Read the model definition and answer for the solid it produces. Units are mm, in the model's axes. Face numbers are marked on the shaded views. A direction names the side the tool comes from. Coordinates: 2 decimals unless noted, no trailing zeros. Loops run counter-clockwise (first coordinate to the right, second up) from the corner with the lowest first, then second, coordinate; pieces in that order, holes last. Notation, with made-up numbers: (22, 15.5) -> (59, 15.5) arc R17 cw to (59, 21.5) -> close; hole circle Ø6 at (0, 86.25). An arc over 180 degrees is marked (long way). Answer in a Markdown table with one row per item.
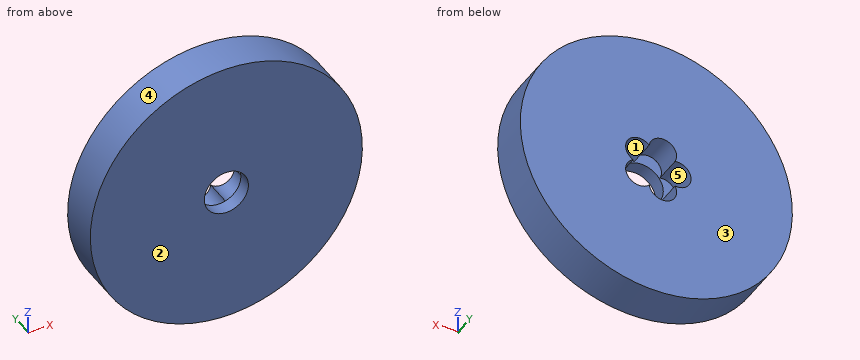
```python
from build123d import *

# Parameters (mm, degrees)
SKETCH1_R           = 92.5
BOSS_EXTRUDE1_DEPTH = 28
SKETCH2_R           = 15
CUT_EXTRUDE1_DEPTH  = 134.777800849
SKETCH3_R           = 9.366362932
CUT_EXTRUDE2_DEPTH  = 18.658456
CIRPATTERN1_START   = 9.341543819
CIRPATTERN1_DEPTH   = 18.658456181


# Read off the part's stored shape, not the designer's step: CirPattern1
with BuildPart() as part:
    # Sketch1 → Boss-Extrude1 (new body)
    with BuildSketch(Plane(origin=(0, 0, 0), x_dir=(1, 0, 0), z_dir=(0, 1, 0))):
        with Locations(Location((0, 0, 0), (0, 0, 270))):
            Circle(SKETCH1_R)
    extrude(amount=BOSS_EXTRUDE1_DEPTH)

    # Sketch2 → Cut-Extrude1 (cut, through all)
    with BuildSketch(Plane(origin=(0, 0, 0), x_dir=(1, 0, 0), z_dir=(0, 1, 0))):
        with Locations(Location((0, 0, 0), (0, 0, 270))):
            Circle(SKETCH2_R)
    extrude(amount=CUT_EXTRUDE1_DEPTH, mode=Mode.SUBTRACT)

    # Sketch3 → Cut-Extrude2 (cut)
    with BuildSketch(Plane(origin=(0, 28, 0), x_dir=(1, 0, 0), z_dir=(0, 1, 0))):
        with Locations((-14.249853525, 0)):
            Circle(SKETCH3_R)
    extrude(amount=-CUT_EXTRUDE2_DEPTH, mode=Mode.SUBTRACT)

    # CirPattern1 outline → CirPattern1 (cut)
    with BuildSketch(Plane(origin=(0, 0, 0), x_dir=(1, 0, 0), z_dir=(0, 1, 0)).offset(CIRPATTERN1_START)):
        with BuildLine():
            ThreePointArc((-11.941511199, -9.077461665), (-12.328101946, -9.167094711), (-12.718142529, -9.240271425))
            ThreePointArc((-12.718142529, -9.240271425), (-7.297812228, -22.460356552), (4.857898172, -14.951073231))
            ThreePointArc((4.857898172, -14.951073231), (19.105920457, -13.881263749), (15.720488714, 0))
            ThreePointArc((15.720488714, 0), (19.105920457, 13.881263749), (4.857898172, 14.951073231))
            ThreePointArc((4.857898172, 14.951073231), (-7.297812228, 22.460356552), (-12.718142529, 9.240271425))
            ThreePointArc((-12.718142529, 9.240271425), (-12.328101946, 9.167094711), (-11.941511199, 9.077461665))
            ThreePointArc((-11.941511199, 9.077461665), (15, 0), (-11.941511199, -9.077461665))
        make_face()
    extrude(amount=CIRPATTERN1_DEPTH, mode=Mode.SUBTRACT)


solid = part.part
```
1. A cutting plane is placed at A-A on x = 0. Give the vertices of the cut face in (y, z).
A:
| item | result |
|---|---|
| outline | (0, -92.5) -> (28, -92.5) -> (28, -21.82) -> (9.34, -21.82) -> (9.34, -15) -> (0, -15) -> close; (0, 15) -> (9.34, 15) -> (9.34, 21.82) -> (28, 21.82) -> (28, 92.5) -> (0, 92.5) -> close |
2. Find the intervals of material crossed by probe 1 along X at (y, z) = (4.25, 0); probe 2 along X at (y, z) = (13.5, 11); probe 3 along Z at (x, y) = (13, 9), in increasing order.
A:
| item | result |
|---|---|
| probe 1 | x = -92.5 to -15, 15 to 92.5 |
| probe 2 | x = -91.84 to -13.42, 20.52 to 91.84 |
| probe 3 | z = -91.58 to -7.48, 7.48 to 91.58 |
3. A tool of negligible diameter and unlimited length cuts with its end or side. For the marked faces 1 and 2, from which of +Z, -Z, +X, -X, +Y, -Y can it reach the whole face along a straight path? Write none if from no direction.
A:
| item | result |
|---|---|
| face 1 | +Y |
| face 2 | +Z, -Z, +X, -X, -Y |
4. A cutting plane is placed at B-B on z = -3. Give the vertices of the cut face in (x, y), and give its area (3 significant figures).
A:
| item | result |
|---|---|
| outline | (-92.45, 0) -> (-14.7, 0) -> (-14.7, 9.34) -> (-23.12, 9.34) -> (-23.12, 28) -> (-92.45, 28) -> close; (14.7, 0) -> (92.45, 0) -> (92.45, 28) -> (19.2, 28) -> (19.2, 9.34) -> (14.7, 9.34) -> close |
| area | 4,110 mm2 |
5. A cutting plane is placed at D-D on x = 57. Give the vertices of the cut face in (y, z), and give its area (3 significant figures).
A:
| item | result |
|---|---|
| outline | (0, -72.85) -> (28, -72.85) -> (28, 72.85) -> (0, 72.85) -> close |
| area | 4,080 mm2 |
6. The mould has two halves that part along X. Classify the marked faces 3, 4 and 5: pulls with the +X half, pulls with the -X half, needs draft (parallel to the pull), parting line crosses it, or undercut.
A:
| item | result |
|---|---|
| face 3 | needs draft |
| face 4 | parting line crosses it |
| face 5 | undercut |
7. Given pin 1 Ø5 at (x, y) = (-64.5, 12.5) entering from -Z; pin 2 Ø2 at (x, y) = (17.5, 13.5) entering from +Z; pin 3 Ø1 at (x, y) = (6, 11) entering from -Z, each flat-ended and moving along its own axis, determine where each tip first touches the part or whether it passes through.
A:
| item | result |
|---|---|
| pin 1 | stops at z = -68.65 |
| pin 2 | stops at z = 91.02 |
| pin 3 | stops at z = -92.34 |
8. A cutting plane is placed at C-C on y = 11.75. Give the vertices of the cut face in (x, z), and give its area (3 significant figures).
A:
| item | result |
|---|---|
| outline | circle Ø185 at (0, 0); hole (-12.72, -9.24) arc R9.37 ccw (long way) to (4.86, -14.95) arc R9.37 ccw (long way) to (15.72, 0) arc R9.37 ccw (long way) to (4.86, 14.95) arc R9.37 ccw (long way) to (-12.72, 9.24) arc R9.37 ccw (long way) to start |
| area | 25,500 mm2 |
